```python
from build123d import *

# Parameters (mm, degrees)
SKETCH1_W           = 110
SKETCH1_H           = 110
BOSS_EXTRUDE1_DEPTH = 3
CUT_EXTRUDE1_DEPTH  = 10
CUT_EXTRUDE2_DEPTH  = 10
CUT_EXTRUDE3_DEPTH  = 10
FILLET1_R           = 5
SKETCH5_W           = 3
SKETCH5_H           = 20
SKETCH5_H_2         = 21.80661572
CUT_EXTRUDE4_DEPTH  = 3


with BuildPart() as part:
    # Sketch1 → Boss-Extrude1 (new body)
    with BuildSketch(Plane(origin=(0, 0, 0), x_dir=(0, 0, -1), z_dir=(1, 0, 0))):
        with Locations((55, -55)):
            Rectangle(SKETCH1_W, SKETCH1_H)
    extrude(amount=BOSS_EXTRUDE1_DEPTH)

    # Sketch2 → Cut-Extrude1 (cut)
    with BuildSketch(Plane(origin=(3, 0, 0), x_dir=(0, 0, -1), z_dir=(1, 0, 0))):
        with BuildLine():
            Line((26.778826095, -55.88152198), (29.40983865, -43.907010607))
            Line((29.40983865, -43.907010607), (9.875793007, -39.61503428))
            ThreePointArc((9.875793007, -39.61503428), (13.975453089, -32.950696648), (21.500097135, -30.80585613))
            ThreePointArc((21.500097135, -30.80585613), (62.897028718, -50.033250753), (91.384991868, -85.69604094))
            ThreePointArc((91.384991868, -85.69604094), (92.19972432, -90.586303718), (90.744288497, -95.325519429))
            Line((90.744288497, -95.325519429), (80.864556452, -107.820216293))
            Line((80.864556452, -107.820216293), (79.448988361, -110))
            Line((79.448988361, -110), (0, -110))
            Line((0, -110), (0, -69.727563309))
            Line((0, -69.727563309), (3.14357432, -66.357579934))
            ThreePointArc((3.14357432, -66.357579934), (4.130318316, -65.093257024), (4.613767896, -63.564057026))
            Line((4.613767896, -63.564057026), (24.14781354, -67.856033353))
            Line((24.14781354, -67.856033353), (26.778826095, -55.88152198))
        make_face()
    extrude(amount=-CUT_EXTRUDE1_DEPTH, mode=Mode.SUBTRACT)

    # Sketch3 → Cut-Extrude2 (cut)
    with BuildSketch(Plane(origin=(3, 0, 0), x_dir=(0, 0, -1), z_dir=(1, 0, 0))):
        Polygon((26.778826095, -55.88152198), (0, -49.997738878), (0, -22.392653141), (110, -2.392653141), (110, 0), (0, 0), (-15.446531008, -25.16825398), (-7.23919485, -70.308602848), (0, -69.727563309), (28.662258875, -73.688951531), (31.123409687, -55.88152198), align=None)
    extrude(amount=-CUT_EXTRUDE2_DEPTH, mode=Mode.SUBTRACT)

    # Sketch4 → Cut-Extrude3 (cut)
    with BuildSketch(Plane(origin=(3, 0, 0), x_dir=(0, 0, -1), z_dir=(1, 0, 0))):
        Polygon((92.19972432, -90.586303718), (110, -90.586303718), (115.849676558, -112.577173273), (92.19972432, -118.868173766), (68.110039343, -115.722673519), (77.620590823, -97.250185318), align=None)
    extrude(amount=-CUT_EXTRUDE3_DEPTH, mode=Mode.SUBTRACT)

    # Fillet1
    fillet1_edges = [part.edges().sort_by_distance(p)[0] for p in [
        (1.5, -90.586303718, -92.19972432),
        (1.5, -90.586303718, -110),
        (1.5, -43.907010607, -29.40983865),
        (1.5, -55.88152198, -26.778826095),
        (1.5, -2.392653141, -110),
        (1.5, -22.392653141, 0),
        (1.5, -49.997738878, 0),
    ]]
    fillet(fillet1_edges, radius=FILLET1_R)

    # Sketch5 → Cut-Extrude4 (cut)
    with BuildSketch(Plane(origin=(0, -21.676088241, -3.941106953), x_dir=(1, 0, 0), z_dir=(0, 0.9838699100999075, 0.17888543819998315))):
        with Locations((1.5, 91.80661572)):
            Rectangle(SKETCH5_W, SKETCH5_H)
        with Locations((1.5, 51.80661572)):
            Rectangle(SKETCH5_W, SKETCH5_H)
        with Locations((1.5, 10.90330786)):
            Rectangle(SKETCH5_W, SKETCH5_H_2)
    extrude(amount=-CUT_EXTRUDE4_DEPTH, mode=Mode.SUBTRACT)


solid = part.part
```
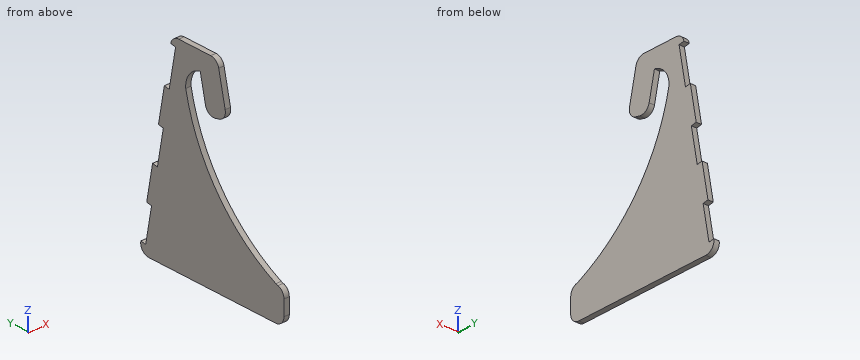
Check sheet for the modelled part. Datum: model origin and axes. Units: mm. Give positions to 0.01 mm unless a question says otherwise; leave off trailing zeros. Write each loop counter-clockwise with the first axis right and the second up, starting at its lowest first coordinate (ties: lowest second). Pieces come first, ordered by that corner, then holes.
Item 1: Scan lines: L1, parallel to Y at x = 2.55, z = -18; L2, parallel to Y at x = 0.5, z = -15.5; L3, parallel to Z at x = 1.2, y = -67. Record each from-to range of solid material in increasing order.
Item 2: Cross-section at C-C (y = -36.5). Enter the section's corners in (x, z), and give its area (3 significant figures).
Item 3: Cross-section at A-A (z = -16.5). Enter the section's corners in (x, y).
Item 4: Cross-section at B-B (x = 2.25). Enter the section's corners in (y, z) (1 decimal), and give its area (3 significant figures).
Item 5: Cross-section at D-D (y = -64.5). Enter the section's corners in (x, z).
Report:
1. L1: y = -53.95 to -41.4, -31.05 to -22.17
1. L2: y = -53.4 to -40.85, -31.98 to -22.62
1. L3: z = -110 to -79.83
2. outline: (0, -110) - (3, -110) - (3, -39.88) - (0, -39.88) - close; (0, -10.96) - (3, -10.96) - (3, 0) - (0, 0) - close
2. area: 243 mm2
3. outline: (0, -53.62) - (3, -53.62) - (3, -41.07) - (0, -41.07) - close; (0, -31.53) - (3, -31.53) - (3, -22.44) - (0, -22.44) - close
4. outline: (-90.6, -105) arc R5 ccw to (-85.6, -110) - (-8.4, -110) arc R5 ccw to (-3.5, -104.1) - (-6.4, -104.6) - (-10, -85) - (-7, -84.4) - (-10.6, -64.8) - (-13.6, -65.3) - (-17.1, -45.6) - (-14.2, -45.1) - (-17.8, -25.4) - (-20.7, -25.9) - (-24.6, -4.5) - (-21.7, -3.9) arc R5 ccw to (-26.6, 0) - (-46, 0) arc R5 ccw to (-50.9, -3.9) - (-54.8, -21.9) arc R5 ccw to (-51, -27.9) - (-48.8, -28.3) arc R5 ccw to (-42.8, -24.5) - (-39.6, -9.9) arc R10.8 cw to (-30.8, -21.5) arc R99.7 cw to (-85.7, -91.4) arc R10.8 cw to (-86.9, -91.8) arc R5 ccw to (-90.6, -96.6) - close
4. area: 4,660 mm2
5. outline: (0, -110) - (3, -110) - (3, -77.81) - (0, -77.81) - close
